Read the model definition and answer for the solid it produces. Units are mm, in the model's axes. A direction names the side the tool comes from. Coordinates: 2 decimals unless noted, no trailing zeros. Write each loop counter-clockwise with the first axis right and the second up, starting at its lowest first coordinate (ties: lowest second). Pieces come first, ordered by that corner, then holes. Notation, with made-up numbers: (56, -14) - (86, -14) arc R23 cw to (86, 4) - close; hole circle Ø10 at (-24, -17). An arc over 180 degrees is marked (long way). Use a Markdown table: item, result.
from build123d import *

# Parameters (mm, degrees)
F1_DEPTH      = 3.175
F1_DEPTH_BACK = 3.175
F3_DEPTH      = 25.4
F3_DEPTH_BACK = 25.4
F5_DEPTH      = 25.4
F5_DEPTH_BACK = 25.4


with BuildPart() as f1:
    # F0 (on Front) → F1 (new body, two sides)
    with BuildSketch(Plane.XZ) as f1_sk:
        with BuildLine():
            Line((-7.62, 0), (0, 0))
            Line((0, 0), (0, 38.1))
            Line((0, 38.1), (-6.35, 38.1))
            Line((-6.35, 38.1), (-15.9218513609, 0.3163762068))
            ThreePointArc((-15.9218513609, 0.3163762068), (-15.8760784336, 0.0979992893), (-15.6756294918, 0))
            Line((-15.6756294918, 0), (-13.97, 0))
            Line((-13.97, 0), (-13.97, -6.096))
            ThreePointArc((-13.97, -6.096), (-13.8956051224, -6.2756051224), (-13.716, -6.35))
            Line((-13.716, -6.35), (-7.874, -6.35))
            ThreePointArc((-7.874, -6.35), (-7.6943948776, -6.2756051224), (-7.62, -6.096))
            Line((-7.62, -6.096), (-7.62, 0))
        make_face()
        with BuildLine():
            Line((0, 38.1), (0, 0))
            Line((0, 0), (7.62, 0))
            Line((7.62, 0), (7.62, -6.096))
            ThreePointArc((7.62, -6.096), (7.6943948776, -6.2756051224), (7.874, -6.35))
            Line((7.874, -6.35), (13.716, -6.35))
            ThreePointArc((13.716, -6.35), (13.8956051224, -6.2756051224), (13.97, -6.096))
            Line((13.97, -6.096), (13.97, 0))
            Line((13.97, 0), (15.6756294918, 0))
            ThreePointArc((15.6756294918, 0), (15.8760784336, 0.0979992893), (15.9218513609, 0.3163762068))
            Line((15.9218513609, 0.3163762068), (6.35, 38.1))
            Line((6.35, 38.1), (0, 38.1))
        make_face()
        with BuildLine():
            Line((-6.35, 38.1), (0, 38.1))
            Line((0, 38.1), (6.35, 38.1))
            Line((6.35, 38.1), (12.0015, 38.1))
            Line((12.0015, 38.1), (12.0015, 41.4839549129))
            Line((12.0015, 41.4839549129), (7.3365180277, 41.4839549129))
            ThreePointArc((7.3365180277, 41.4839549129), (7.1198722569, 41.6053630202), (7.1103332026, 41.8535249129))
            Line((7.1103332026, 41.8535249129), (12.6253100407, 52.6470186525))
            ThreePointArc((12.6253100407, 52.6470186525), (12.6518210481, 52.7882949989), (12.5974039021, 52.9213386525))
            Line((12.5974039021, 52.9213386525), (0.1982786864, 68.4078410832))
            ThreePointArc((0.1982786864, 68.4078410832), (0, 68.5030910832), (-0.1982786864, 68.4078410832))
            Line((-0.1982786864, 68.4078410832), (-12.5974039021, 52.9213386525))
            ThreePointArc((-12.5974039021, 52.9213386525), (-12.6518210481, 52.7882949989), (-12.6253100407, 52.6470186525))
            Line((-12.6253100407, 52.6470186525), (-7.1103332026, 41.8535249129))
            ThreePointArc((-7.1103332026, 41.8535249129), (-7.1198722569, 41.6053630202), (-7.3365180277, 41.4839549129))
            Line((-7.3365180277, 41.4839549129), (-12.0015, 41.4839549129))
            Line((-12.0015, 41.4839549129), (-12.0015, 38.1))
            Line((-12.0015, 38.1), (-6.35, 38.1))
        make_face()
        with BuildLine():
            Line((-13.7196155367, 38.1), (-12.0015, 38.1))
            Line((-12.0015, 38.1), (-12.0015, 41.4839549129))
            Line((-12.0015, 41.4839549129), (-13.9330163108, 38.4917538008))
            ThreePointArc((-13.9330163108, 38.4917538008), (-13.9426687427, 38.2324958136), (-13.7196155367, 38.1))
        make_face()
        with BuildLine():
            Line((12.0015, 41.4839549129), (12.0015, 38.1))
            Line((12.0015, 38.1), (13.7196155367, 38.1))
            ThreePointArc((13.7196155367, 38.1), (13.9426687427, 38.2324958136), (13.9330163108, 38.4917538008))
            Line((13.9330163108, 38.4917538008), (12.0015, 41.4839549129))
        make_face()
    extrude(amount=F1_DEPTH)
    extrude(f1_sk.sketch, amount=-F1_DEPTH_BACK)

    # F2 (on Front) → F3 (cut, two sides)
    with BuildSketch(Plane.XZ) as f3_sk:
        Polygon((-3.1575310771, 55.0611501542), (-7.7323545702, 64.2502829432), (-9.8524354398, 61.3006092608), (-4.4139670208, 54.1107691824), align=None)
    extrude(amount=-F3_DEPTH, mode=Mode.SUBTRACT)
    extrude(f3_sk.sketch, amount=F3_DEPTH_BACK, mode=Mode.SUBTRACT)

    # F4 (on Front) → F5 (cut, two sides)
    with BuildSketch(Plane.XZ) as f5_sk:
        Polygon((1.778, 5.715), (-1.778, 5.715), (-1.778, 4.7625), (-3.81, 4.7625), (-3.81, 2.2225), (-1.778, 2.2225), (-1.778, 0), (1.778, 0), (1.778, 2.2225), (3.81, 2.2225), (3.81, 4.7625), (1.778, 4.7625), align=None)
    extrude(amount=F5_DEPTH, mode=Mode.SUBTRACT)
    extrude(f5_sk.sketch, amount=-F5_DEPTH_BACK, mode=Mode.SUBTRACT)


solid = f1.part
(1) Each of these flat-tipped pins is pushed along its axis until it touches: P1, Ø3, axis at y = 1.5, z = 33, coming from the +X side; P2, Ø0.8, axis at y = -1.5, z = 5, coming from the -X side; P3, Ø1.4, axis at x = 14.5, y = -0.5, coming from the -Z side; P4, Ø1.5, axis at x = -10, z = 60.5, coming from the +Y side. Where does it stop, or does it pass through?
Report:
| item | result |
|---|---|
| P1 | stops at x = 8.02 |
| P2 | stops at x = -14.84 |
| P3 | stops at z = -6.34 |
| P4 | passes through |
(2) The mould has two halves that part along Z. Classify faces 1 (the flat face through (-1.778, 0, 1)), 2 (the flat face through (3, 0, 4.762)), 3 (the flat face through (5, 0, 0)): pulls with the +Z half, pulls with the -Z half, needs draft (parallel to the pull), parting line crosses it, or undercut.
Report:
| item | result |
|---|---|
| face 1 | needs draft |
| face 2 | undercut |
| face 3 | pulls with the -Z half |
(3) A cutting plane is placed at D-D, the plane z = 59.5. Write down the section's boundary in (x, y) (3 decimals), and give its area (3 significant figures).
Report:
| item | result |
|---|---|
| outline | (-5.367, -3.175) - (7.33, -3.175) - (7.33, 3.175) - (-5.367, 3.175) - close |
| area | 80.6 mm² |
(4) A cutting plane is placed at A-A, the plane z = -1. Write down the section's boundary in (x, y) (3 decimals).
Report:
| item | result |
|---|---|
| outline | (-13.97, -3.175) - (-7.62, -3.175) - (-7.62, 3.175) - (-13.97, 3.175) - close; (7.62, -3.175) - (13.97, -3.175) - (13.97, 3.175) - (7.62, 3.175) - close |
(5) A cutting plane is placed at B-B, the plane x = -11. Count the separate pieces of the cut face and the enclosed holes in it, and give its area (3 significant figures).
Report:
| item | result |
|---|---|
| separate pieces | 3 |
| enclosed holes | 0 |
| area | 222 mm² |
(6) For faces 4 (the flat face through (-3.81, 0, 4)), 5 (the flat face through (-10, 0, 41.484)), 6 (the flat face through (15, 0, 0)), 7 (the flat face through (10, 0, 38.1)), determine the directions among +Z, -Z, +X, -X, +Y, -Y from which every point of the face is accessible in a straight line to the end or side of a thin tool.
Report:
| item | result |
|---|---|
| face 4 | +Y, -Y |
| face 5 | -X, +Y, -Y |
| face 6 | -Z, +X, +Y, -Y |
| face 7 | +X, +Y, -Y |
(7) Straight lines are drawn through the part: L1, parallel to X at y = 0, z = -0.5; L2, parallel to Z at x = 0, y = -2 (3 decimals); L3, parallel to X at y = 2, z = 5. For each, find the intervals that lie inside material, in ascending order.
Report:
| item | result |
|---|---|
| L1 | x = -13.97 to -7.62, 7.62 to 13.97 |
| L2 | z = 5.715 to 68.503 |
| L3 | x = -14.74 to -1.78, 1.78 to 14.74 |
